Work out the finished part from the listing and answer in its coordinate system (mm). Face numbers are marked on the shaded views. Round coordinates to 2 decimals unless told otherwise and drop trailing zeros. Order: outer loops, then holes, each group sorted by start corner. A loop starts at its lowest first (then second) coordinate and runs counter-clockwise, first axis right, second up.
from build123d import *

# Parameters (mm, degrees)
SKETCH_1_R          = 25.25
EXTRUDE_1_DEPTH     = 5
SKETCH_2_R          = 23.85
EXTRUDE_2_DEPTH     = 1
CHAMFER_2_SIZE      = 0.5
CUT_EXTRUDE_1_DEPTH = 1
SKETCH_4_R          = 26.25
SKETCH_4_R_2        = 25.25
EXTRUDE_3_DEPTH     = 1
SKETCH_5_R          = 2.5
EXTRUDE_4_DEPTH     = 1
SKETCH_6_R          = 1.65
CUT_EXTRUDE_2_DEPTH = 3.5
FILLET_2_R          = 1


with BuildPart() as part:
    # 草图1 → 凸台-拉伸1 (new body)
    with BuildSketch(Plane.XY):
        with BuildLine():
            Line((-36, 29), (36, 29))
            ThreePointArc((36, 29), (40.242640687, 27.242640687), (42, 23))
            Line((42, 23), (42, -23))
            ThreePointArc((42, -23), (40.242640687, -27.242640687), (36, -29))
            Line((36, -29), (-36, -29))
            ThreePointArc((-36, -29), (-40.242640687, -27.242640687), (-42, -23))
            Line((-42, -23), (-42, 23))
            ThreePointArc((-42, 23), (-40.242640687, 27.242640687), (-36, 29))
        make_face()
        Circle(SKETCH_1_R, mode=Mode.SUBTRACT)
    extrude(amount=EXTRUDE_1_DEPTH)

    # 草图2 → 凸台-拉伸2 (add)
    with BuildSketch(Plane.XY.offset(5)):
        with BuildLine():
            Line((36, 29), (-36, 29))
            ThreePointArc((-36, 29), (-40.242640687, 27.242640687), (-42, 23))
            Line((-42, 23), (-42, -23))
            ThreePointArc((-42, -23), (-40.242640687, -27.242640687), (-36, -29))
            Line((-36, -29), (36, -29))
            ThreePointArc((36, -29), (40.242640687, -27.242640687), (42, -23))
            Line((42, -23), (42, 23))
            ThreePointArc((42, 23), (40.242640687, 27.242640687), (36, 29))
        make_face()
        Circle(SKETCH_2_R, mode=Mode.SUBTRACT)
    extrude(amount=EXTRUDE_2_DEPTH)

    # 倒角2
    chamfer_2_edges = [part.edges().sort_by_distance(p)[0] for p in [
        (-23.85, 0, 5),
    ]]
    chamfer(chamfer_2_edges, length=CHAMFER_2_SIZE)

    # 草图3 → 切除-拉伸1 (cut)
    with BuildSketch(Plane.XY.offset(6)):
        with BuildLine():
            Line((36, 27), (-36, 27))
            ThreePointArc((-36, 27), (-38.828427125, 25.828427125), (-40, 23))
            Line((-40, 23), (-40, -23))
            ThreePointArc((-40, -23), (-38.828427125, -25.828427125), (-36, -27))
            Line((-36, -27), (36, -27))
            ThreePointArc((36, -27), (38.828427125, -25.828427125), (40, -23))
            Line((40, -23), (40, 23))
            ThreePointArc((40, 23), (38.828427125, 25.828427125), (36, 27))
        make_face()
    extrude(amount=-CUT_EXTRUDE_1_DEPTH, mode=Mode.SUBTRACT)

    # 草图4 → 凸台-拉伸3 (add)
    with BuildSketch(Plane.XY.offset(5)):
        Circle(SKETCH_4_R)
        Circle(SKETCH_4_R_2, mode=Mode.SUBTRACT)
    extrude(amount=EXTRUDE_3_DEPTH)

    # 草图5 → 凸台-拉伸4 (add)
    with BuildSketch(Plane.XY.offset(5)):
        with Locations((36, 23)):
            Circle(SKETCH_5_R)
        with Locations(Location((36, -23, 0), (0, 0, 180))):
            Circle(SKETCH_5_R)
        with Locations(Location((-36, 23, 0), (0, 0, 180))):
            Circle(SKETCH_5_R)
        with Locations((-36, -23)):
            Circle(SKETCH_5_R)
    extrude(amount=EXTRUDE_4_DEPTH)

    # 草图6 → 切除-拉伸2 (cut)
    with BuildSketch(Plane.XY.offset(6)):
        with Locations((36, 23)):
            Circle(SKETCH_6_R)
        with Locations(Location((36, -23, 0), (0, 0, 180))):
            Circle(SKETCH_6_R)
        with Locations(Location((-36, 23, 0), (0, 0, 180))):
            Circle(SKETCH_6_R)
        with Locations((-36, -23)):
            Circle(SKETCH_6_R)
    extrude(amount=-CUT_EXTRUDE_2_DEPTH, mode=Mode.SUBTRACT)

    # 圆角2
    fillet_2_edges = [part.edges().sort_by_distance(p)[0] for p in [
        (-42, 0, 0),
        (-40.242640687, 27.242640687, 0),
        (0, 29, 0),
        (40.242640687, 27.242640687, 0),
        (-25.25, 0, 0),
        (42, 0, 0),
        (40.242640687, -27.242640687, 0),
        (0, -29, 0),
        (-40.242640687, -27.242640687, 0),
    ]]
    fillet(fillet_2_edges, radius=FILLET_2_R)


solid = part.part
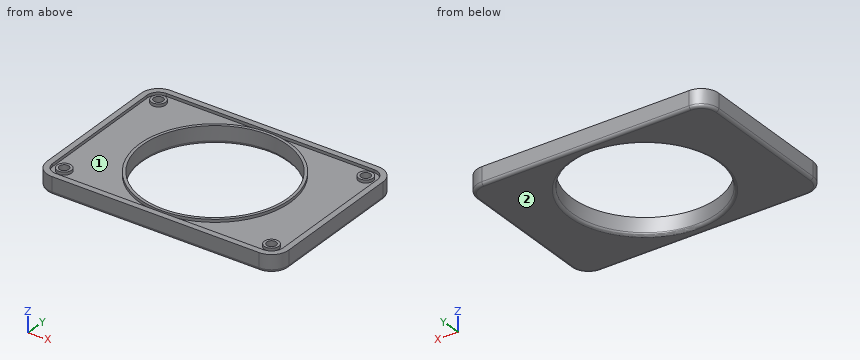
Item 1: Find the intervals of material crossed by line 1 along Y through (x, z) = (36, 3.9); line 2 along Y through (x, z) = (0, 4.1); line 3 along X through (y, z) = (17.5, 5.35), in increasing order.
Item 2: Given pin 1 (1 mm diameter, centred on x = -36, y = 22.5, fed in from +Z); pin 2 (10 mm diameter, centred on x = -19, y = -6.5, fed in from +Z), each flat-ended and moving along its own axis, determine where each tip first touches the part or whether it passes through.
Item 3: Find section A-A (x = 0). Write down the section's boundary in (y, z).
Item 4: Find section B-B (z = 4.15). Write down the section's boundary in (x, y), plus the area to 3 significant figures.
Item 5: Find section C-C (y = 0). Write down the section's boundary in (x, z), plus the area to 3 significant figures.
Item 6: For a pull along X with two mould halves and no side action, classify the marked faces 1 and 2 as released by +X, released by -X, zero draft, split by the parting line, or undercut.
Model answer:
1. line 1: y = -29 to -24.65, -21.35 to 21.35, 24.65 to 29
1. line 2: y = -29 to -25.25, 25.25 to 29
1. line 3: x = -42 to -40, -19.57 to -18.2, 18.2 to 19.57, 40 to 42
2. pin 1: stops at z = 2.5
2. pin 2: passes through
3. outline: (-29, 1) arc R1 ccw to (-28, 0) - (-26.25, 0) arc R1 ccw to (-25.25, 1) - (-25.25, 6) - (-26.25, 6) - (-26.25, 5) - (-27, 5) - (-27, 6) - (-29, 6) - close; (25.25, 1) arc R1 ccw to (26.25, 0) - (28, 0) arc R1 ccw to (29, 1) - (29, 6) - (27, 6) - (27, 5) - (26.25, 5) - (26.25, 6) - (25.25, 6) - close
4. outline: (-42, -23) arc R6 ccw to (-36, -29) - (36, -29) arc R6 ccw to (42, -23) - (42, 23) arc R6 ccw to (36, 29) - (-36, 29) arc R6 ccw to (-42, 23) - close; hole circle Ø3.3 at (-36, -23); hole circle Ø3.3 at (-36, 23); hole circle Ø50.5 at (0, 0); hole circle Ø3.3 at (36, -23); hole circle Ø3.3 at (36, 23)
4. area: 2,800 mm2
5. outline: (-42, 1) arc R1 ccw to (-41, 0) - (-26.25, 0) arc R1 ccw to (-25.25, 1) - (-25.25, 6) - (-26.25, 6) - (-26.25, 5) - (-40, 5) - (-40, 6) - (-42, 6) - close; (25.25, 1) arc R1 ccw to (26.25, 0) - (41, 0) arc R1 ccw to (42, 1) - (42, 6) - (40, 6) - (40, 5) - (26.25, 5) - (26.25, 6) - (25.25, 6) - close
5. area: 173 mm2
6. face 1: undercut
6. face 2: zero draft
